Could you check a few things on this drawing? It's one solid part, dimensions in mm from its lowest x, y, z. A direction names the side the tool comes from. Give positions to 0.01 mm unless a question says otherwise; leave off trailing zeros. Order: outer loops, then holes, each group sorted by start corner. A loop starts at its lowest first (then second) coordinate and runs counter-clockwise, first axis right, second up. Notation, with made-up numbers: M -3.5,46.5 L 49.5,46.5 A14 ccw 49.5,71.5 Z; hole C 62,22.5 d10. An arc over 180 degrees is marked long. Use one line per item in the form item = value.
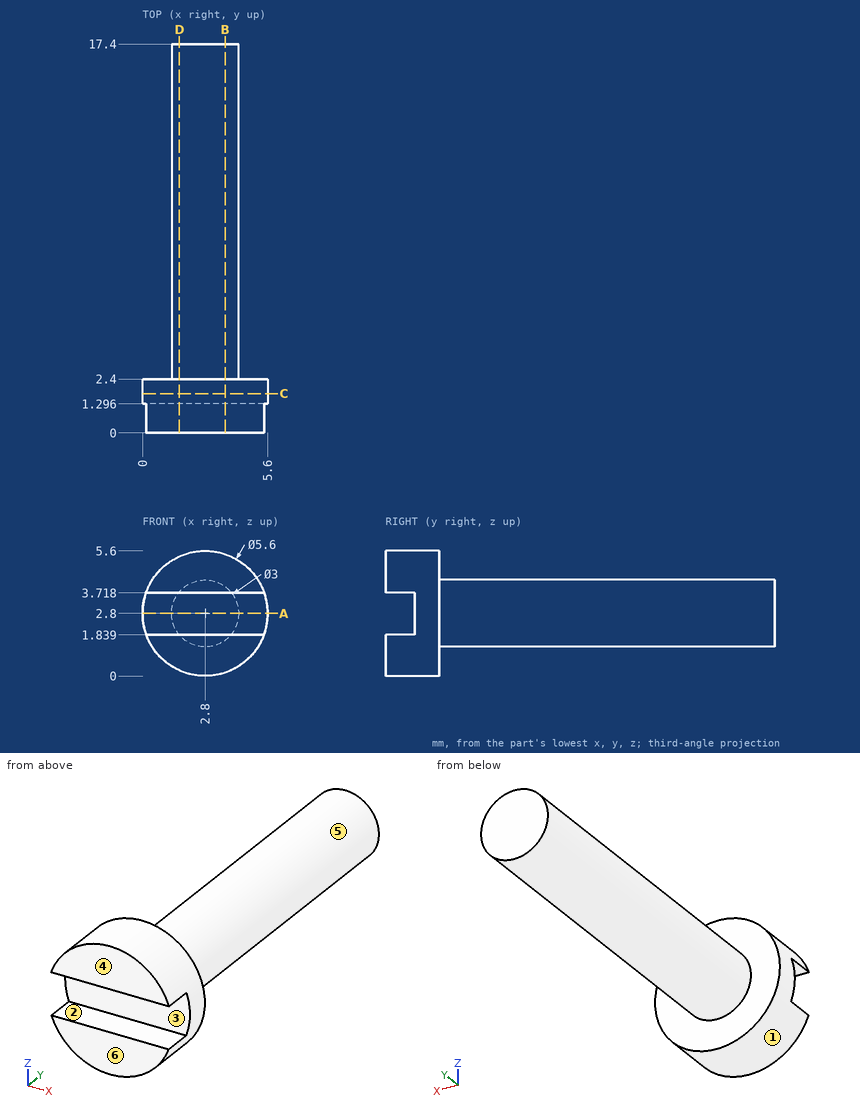
Q1. I want a section at B-B on x = 3.7. Write out the boundary of the cut face in (y, z).
Found:
outline = M 0,0.15 L 2.4,0.15 L 2.4,1.6 L 17.4,1.6 L 17.4,4 L 2.4,4 L 2.4,5.45 L 0,5.45 L 0,3.72 L 1.3,3.72 L 1.3,1.84 L 0,1.84 Z
Q2. Thinking about a two-plate mould opening in Z: for the marked faces 1, 2, 3 and 4, which applies, +Z half, -Z half, draft (parallel to the pull), parting line (faces both ways), or undercut?
Found:
face_1 = parting line
face_2 = undercut
face_3 = undercut
face_4 = draft
Q3. I'm going to push flat-ended pins straight in: pin 1 Ø1.5 at (x, z) = (3.5, 2.5) entering from -Y; pin 2 Ø3 at (x, y) = (1, 9.5) entering from -Z; pin 3 Ø2 at (y, z) = (9, 3.5) entering from +X; pin 4 Ø3 at (y, z) = (6.5, 4.5) entering from -X. Where does each tip first touch, or does it pass through?
Found:
pin_1 = 0
pin_2 = 1.33
pin_3 = 4.3
pin_4 = 1.31
Q4. On a 3-axis mill with a long thin cutter (end or side, diameter ignored), from which of +Z, -Z, +X, -X, +Y, -Y can I reach the whole of each face in a straight line? I mean the marked faces 5 and 6. Say none if no direction works.
Found:
face_5 = +Y
face_6 = +Z, -Z, +X, -X, -Y
Q5. I want a section at D-D on x = 1.65. Write out the boundary of the cut face in (y, z).
Found:
outline = M 0,0.25 L 2.4,0.25 L 2.4,1.84 L 17.4,1.84 L 17.4,3.76 L 2.4,3.76 L 2.4,5.35 L 0,5.35 L 0,3.72 L 1.3,3.72 L 1.3,1.84 L 0,1.84 Z
Q6. I want a section at A-A on z = 2.8. Write out the boundary of the cut face in (x, y).
Found:
outline = M 0,1.3 L 5.6,1.3 L 5.6,2.4 L 4.3,2.4 L 4.3,17.4 L 1.3,17.4 L 1.3,2.4 L 0,2.4 Z
Q7. I want a section at C-C on y = 1.75. Write out the boundary of the cut face in (x, z), then the cut area to 3 significant figures.
Found:
outline = C 2.8,2.8 d5.6
area = 24.6 mm²
Q8. I need wall thicknesses on L1, parallel to Y at x = 1.3, z = 4.45; L2, parallel to Y at x = 3.5, z = 1.9; L3, parallel to Z at x = 2.5, y = 11.25. Which ranges of each line are inside material? Lowest first, please.
Found:
L1 = 0 to 2.4
L2 = 1.3 to 17.4
L3 = 1.33 to 4.27
